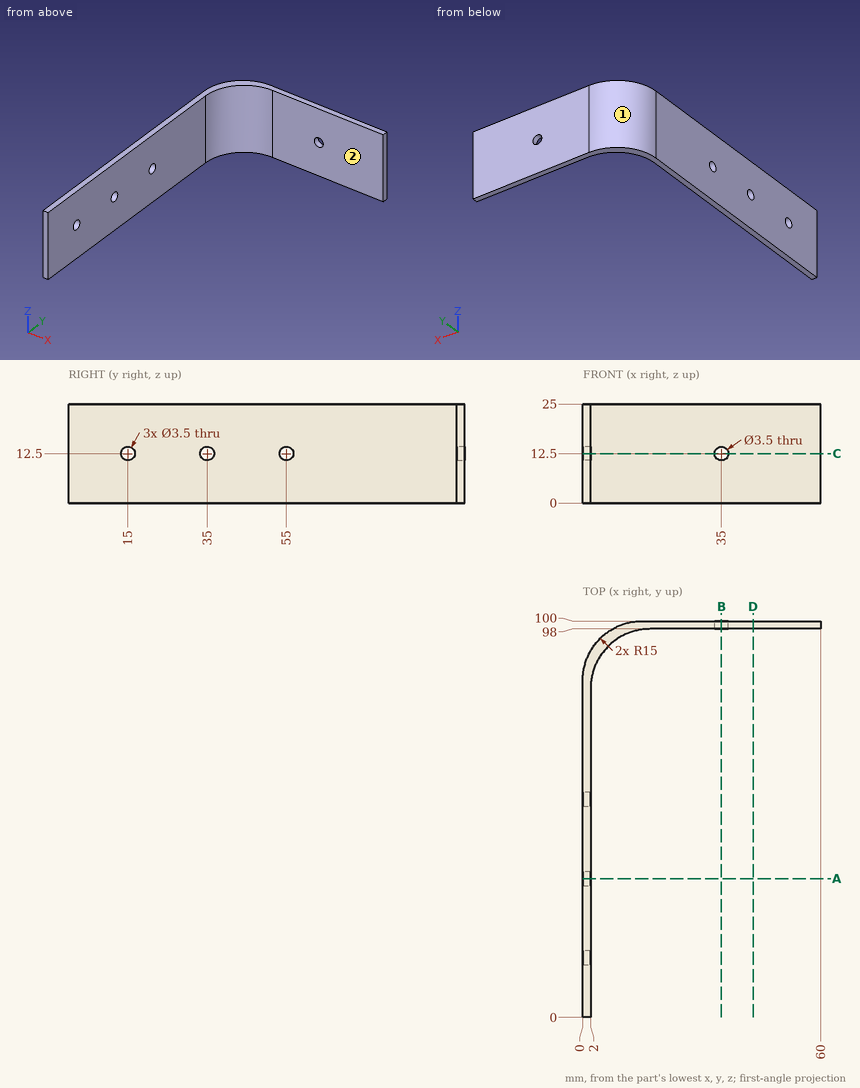
Design review of the part shown in the three views and the two pictorial views. Dimensions are in mm from the part's minimum x, y and z. A direction names the side the tool comes from. Round coordinates to 2 decimals unless told otherwise and drop trailing zeros. Write each loop counter-clockwise with the first axis right and the second up, starting at its lowest first coordinate (ties: lowest second). Pieces come first, ordered by that corner, then holes.
Item 1: Consider section B-B on x = 35. Give the boundary of the cut face in (y, z), and give its area (3 significant figures).
Item 2: Consider section D-D on x = 43. Give the boundary of the cut face in (y, z).
Item 3: For the marked faces 1 and 2, list the 3-axis set-ups (+Z, -Z, +X, -X, +Y, -Y) from which the entire face can be reached by the end or side of a thin tool; tool diameter is ignored.
Item 4: Wall thickness on L1, parallel to Z at x = 1, y = 55; L2, parallel to X at y = 40, z = 6; L3, parallel to Y at x = 36.5, z = 5.5: over which ranges is each line inside the solid? List them lowest first.
Item 5: Consider section C-C on z = 12.5. Give the boundary of the cut face in (x, y).
Item 6: For pin 1 Ø5.5 at (y, z) = (55, 12.5) entering from -X; pin 2 Ø8 at (y, z) = (59, 13) entering from +X; pin 3 Ø5.5 at (x, z) = (35, 12.5) entering from -Y, all flat-tipped, find the tip position at first contact; note any pin that passes through.
Item 7: Consider section A-A on y = 35. Give the boundary of the cut face in (x, z).
Check values:
1. outline: (98, 0) - (100, 0) - (100, 10.75) - (98, 10.75) - close; (98, 14.25) - (100, 14.25) - (100, 25) - (98, 25) - close
1. area: 43.0 mm2
2. outline: (98, 0) - (100, 0) - (100, 25) - (98, 25) - close
3. face 1: +Z, -Z, -X, +Y
3. face 2: +Z, -Z, +X, -Y
4. L1: z = 0 to 10.75, 14.25 to 25
4. L2: x = 0 to 2
4. L3: y = 98 to 100
5. outline: (0, 0) - (2, 0) - (2, 13.25) - (0, 13.25) - close; (0, 16.75) - (2, 16.75) - (2, 33.25) - (0, 33.25) - close; (0, 36.75) - (2, 36.75) - (2, 53.25) - (0, 53.25) - close; (0, 56.75) - (2, 56.75) - (2, 83) arc R15 cw to (17, 98) - (33.25, 98) - (33.25, 100) - (15, 100) arc R15 ccw to (0, 85) - close; (36.75, 98) - (60, 98) - (60, 100) - (36.75, 100) - close
6. pin 1: stops at x = 0
6. pin 2: stops at x = 2
6. pin 3: stops at y = 98
7. outline: (0, 0) - (2, 0) - (2, 10.75) - (0, 10.75) - close; (0, 14.25) - (2, 14.25) - (2, 25) - (0, 25) - close
